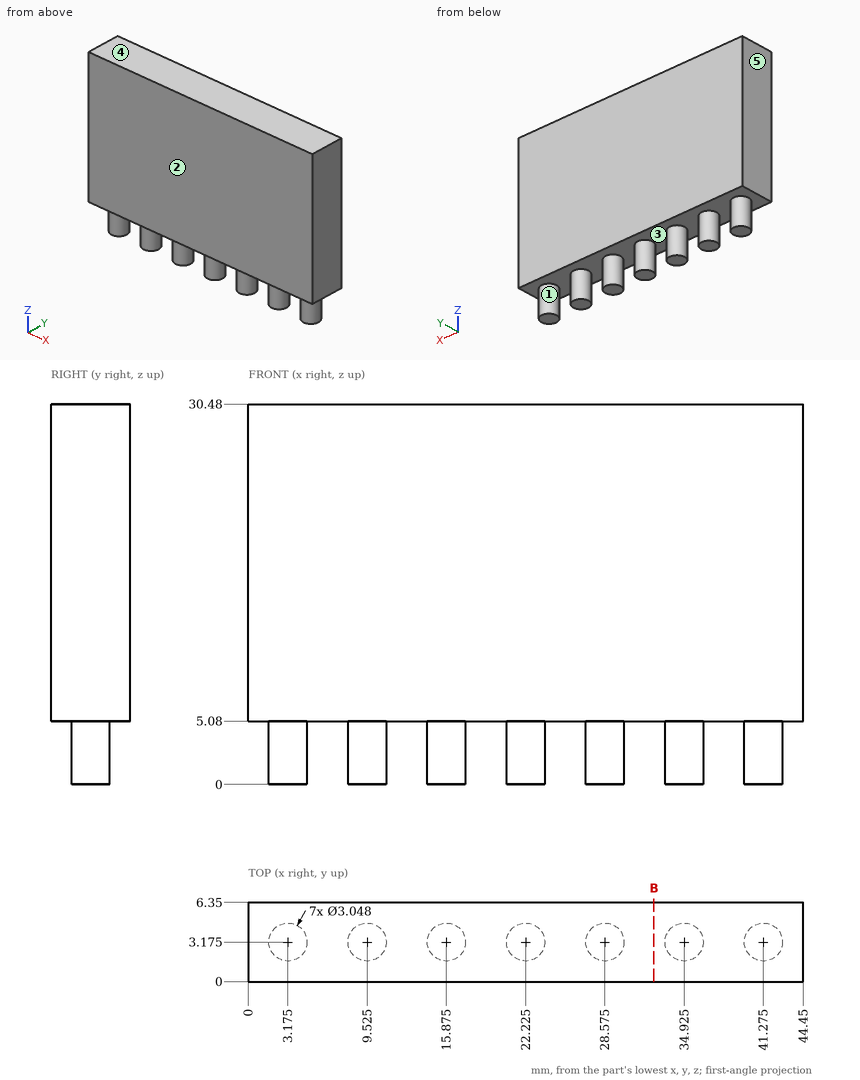
For this review, use the dimensioned drawing (mm, ordinates from the lowest corner) and the shaded views. A direction names the side the tool comes from. Round coordinates to 2 decimals unless told otherwise and drop trailing zeros. Order: outer loops, then holes, each group sorted by start corner. A loop starts at its lowest first (then second) coordinate and runs counter-clockwise, first axis right, second up. Notation, with made-up numbers: (39.25, -32) -> (79.25, -32) arc R15 ccw to (79.25, -14) -> close; hole circle Ø2 at (42, 42). An arc over 180 degrees is marked (long way). One line per item, written item: value. Start each with the question number.
Q1. Wall thickness on line 1 (Z direction, x = 42.5, y = 6.25); line 2 (Y direction, x = 15.5, z = 2): over which ranges is each line inside the solid? List them lowest first.
Q2. Mouldability with a two-part tool opening along X and no side actions: class the marked faces 3, 4 and 5 as released by +X, released by -X, zero draft, split by the parting line, or undercut.
Q3. Clearance check with a flat-ended pin moving along its axis: pin 1 Ø1.5 at (x, y) = (11, 5.5) entering from -Z. State where the tip first meets the part, or that it passes through.
Q4. Take a section at B-B (x = 32.5). Write out the cut boundary in (y, z), and give its area (3 significant figures).
Q5. Machinability: for the marked faces 1 and 2, which of the approach directions +Z, -Z, +X, -X, +Y, -Y give a long, thin tool a straight path to every point of the face, cutting with its end or side? Answer none if there is none.
Reported:
1. line 1: z = 5.08 to 30.48
1. line 2: y = 1.7 to 4.65
2. face 3: undercut
2. face 4: zero draft
2. face 5: released by -X
3. pin 1: stops at z = 5.08
4. outline: (0, 5.08) -> (6.35, 5.08) -> (6.35, 30.48) -> (0, 30.48) -> close
4. area: 161 mm2
5. face 1: -Z
5. face 2: +Z, -Z, +X, -X, -Y
